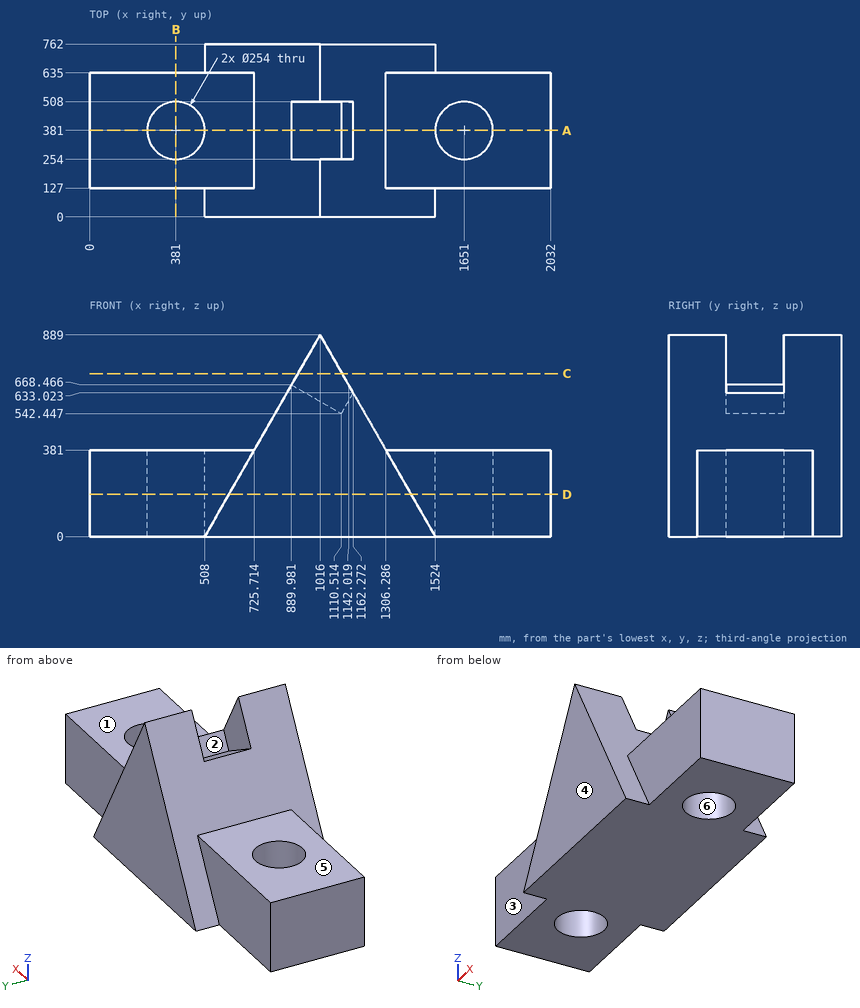
Geometry check sheet. Reference: drawing and pictorial views, mm from the part's lowest x, y, z. A direction names the side the tool comes from. Coordinates: 2 decimals unless noted, no trailing zeros. Loops run counter-clockwise (first coordinate to the right, second up) from the corner with the lowest first, then second, coordinate; pieces in that order, holes last.
1) Sectioned sample at A-A (y = 381). Record the boundary of the cut face in (x, z) (1 decimal), and give its area (3 significant figures).
2) Access from +Z, -Z, +X, -X, +Y, -Y to the whole of each face (thin tool, end or side, straight path). Record for the marked faces 1, 2 and 3.
3) Sectioned sample at C-C (z = 718). Record the boundary of the cut face in (x, y) (1 decimal).
4) Gauge pin test, flat ends, axial feed: pin 1 (4 mm diameter, centred on x = 773.5, y = 364, fed in from +Z) (1 decimal); pin 2 (5 mm diameter, centred on y = 496.5, z = 447.5, fed in from +X) (1 decimal); pin 3 (10 mm diameter, centred on x = 1240, y = 338.5, fed in from +Z). Record the tip position at first contact, or that the pin passes through.
5) Material ranges on probe 1 along Y at (x, z) = (1651, 149); probe 2 along X at (y, z) = (470, 42.5); probe 3 along X at (y, z) = (333, 342.5), recorded low to high.
6) Sectioned sample at B-B (x = 381). Record the boundary of the cut face in (y, z), and give its area (3 significant figures).
7) Release check for a two-part mould opening along Y. For the marked faces 4, 5 and 6 record: released by +Y, released by -Y, zero draft, split by the parting line, or undercut.
8) Sectioned sample at D-D (z = 186). Record the boundary of the cut face in (x, y) (1 decimal).
Check sheet entries:
1. outline: (0, 0) - (254, 0) - (254, 381) - (0, 381) - close; (508, 0) - (1524, 0) - (1524, 381) - (1306.3, 381) - (1162.3, 633) - (1110.5, 542.4) - (890, 668.5) - (725.7, 381) - (508, 381) - close; (1778, 0) - (2032, 0) - (2032, 381) - (1778, 381) - close
1. area: 683,000 mm2
2. face 1: +Z, +X, +Y, -Y
2. face 2: +Z
2. face 3: +Z, -X, -Y
3. outline: (918.3, 0) - (1113.7, 0) - (1113.7, 254) - (918.3, 254) - close; (918.3, 508) - (1113.7, 508) - (1113.7, 762) - (918.3, 762) - close
4. pin 1: stops at z = 468.1
4. pin 2: stops at x = 1269.7
4. pin 3: stops at z = 505.75
5. probe 1: y = 127 to 254, 508 to 635
5. probe 2: x = 0 to 290.4, 471.6 to 1560.4, 1741.6 to 2032
5. probe 3: x = 0 to 263.42, 498.58 to 1533.42, 1768.58 to 2032
6. outline: (127, 0) - (254, 0) - (254, 381) - (127, 381) - close; (508, 0) - (635, 0) - (635, 381) - (508, 381) - close
6. area: 96,800 mm2
7. face 4: released by -Y
7. face 5: zero draft
7. face 6: undercut
8. outline: (0, 127) - (614.3, 127) - (614.3, 0) - (1417.7, 0) - (1417.7, 127) - (2032, 127) - (2032, 635) - (1417.7, 635) - (1417.7, 762) - (614.3, 762) - (614.3, 635) - (0, 635) - close; hole circle Ø254 at (381, 381); hole circle Ø254 at (1651, 381)
